Job drawing, mm, ordinate dimensions from the low corner. One solid piece. Give positions to 0.01 mm unless a question says otherwise; leave off trailing zeros. Order: outer loops, then holes, each group sorted by start corner. A loop starts at its lowest first (then second) coordinate and runs counter-clockwise, first axis right, second up. Notation, with made-up numbers: (-8, 46) - (11, 46) arc R19 ccw to (11, 67) - close; hole circle Ø8 at (82, -25.75). An arc over 180 degrees is marked (long way). One line per item, written item: value.
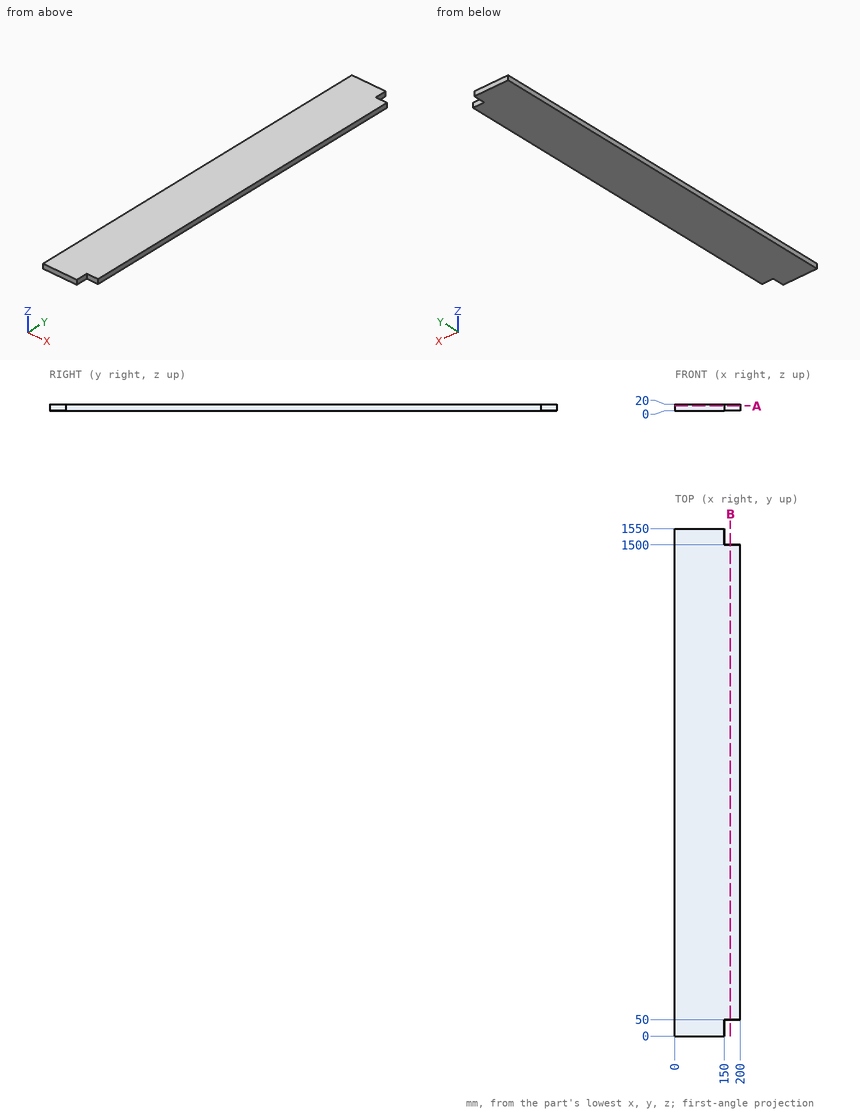
1) Wall check: line 1 along Y through (x, z) = (175.5, 6). Give the ranges that are in metal, low to high. Write a range as [from, to].
Answer:
line 1: y = [50, 1500]
2) Slice it at A-A on z = 14.25. Write the cut outline in (x, y), then the cut area to 3 significant figures.
Answer:
outline: (0, 0) - (150, 0) - (150, 50) - (200, 50) - (200, 1500) - (150, 1500) - (150, 1550) - (0, 1550) - close
area: 305,000 mm2
3) Slice it at B-B on x = 169. Write the cut outline in (y, z).
Answer:
outline: (50, 0) - (1500, 0) - (1500, 20) - (50, 20) - close
4) Drop flat-ended pins along their axis: P1, Ø6, axis at y = 30.5, z = 5.5, coming from the +X side; P2, Ø6, axis at x = 171.5, z = 16, coming from the -Y side. Give the stop position or say it passes through.
Answer:
P1: stops at x = 150
P2: stops at y = 50
